Autodesk Inventor part; units mm, degrees
ref_plane "YZ Plane" through (0, 0, 0) normal (1, 0, 0) x (0, 1, 0)
ref_plane "XZ Plane" through (0, 0, 0) normal (0, 1, 0) x (-1, 0, 0)
ref_plane "XY Plane" through (0, 0, 0) normal (0, 0, 1) x (1, 0, 0)
sketch "Sketch1" plane through (0, 0, 0) normal (0, 1, 0) x (-1, 0, 0)
  line L0 (11, 19.5) -> (-11, 19.5)
  line L1 (-11, 19.5) -> (-11, -19.5)
  line L2 (-11, -19.5) -> (11, -19.5)
  line L3 (11, -19.5) -> (11, 19.5)
  line L4 (11, 19.5) -> (-11, -19.5) construction
  line L5 (-11, 19.5) -> (11, -19.5) construction
  point P0 (0, 0)
  dimension "d0" = 22
  dimension "d1" = 39
extrude "Plate1" add sketch "Sketch1" along normal blind 3
sketch "Sketch2" plane through (0, 3, 0) normal (0, 1, 0) x (1, 0, 0)
  circle A0 centre (0, -12.5) radius 2.1
  line L0 (11, -19.5) -> (11, 19.5)
  line L1 (11, 0) -> (-11, 0)
  line L2 (-11, 19.5) -> (-11, -19.5)
  circle A1 centre (0, 12.5) radius 2.1
  point P0 (0, 0)
  dimension "d3" = 4.2
  dimension "d4" = 12.5
extrude "Cut1" cut sketch "Sketch2" against normal blind 3
equation "\"d5\" = Thickness"
equation "\"d2\" = Thickness"
equation "\"BendRadius\" = Thickness"
equation "\"BendReliefWidth\" = Thickness"
equation "\"BendReliefDepth\" = 0.5 * Thickness"
equation "\"CornerReliefSize\" = 4 * Thickness"
equation "\"MinimumRemnant\" = 2 * Thickness"
equation "\"TransitionRadius\" = BendRadius"
equation "\"JacobiRadiusSize\" = BendRadius"
equation "\"GapSize\" = Thickness"
properties part number "90 graders beslag"
Check sheet for the modelled part. Datum: model origin and axes. Units: mm. Round coordinates to 2 decimals unless told otherwise and drop trailing zeros. Write each loop counter-clockwise with the first axis right and the second up, starting at its lowest first coordinate (ties: lowest second). Pieces come first, ordered by that corner, then holes. Notation, with made-up numbers: (70.5, 37) -> (82.5, 37) arc R21 ccw to (82.5, 51) -> close; hole circle Ø8 at (-8.75, -15). An arc over 180 degrees is marked (long way). Put each result on its own line as item: value.
(1) Sectioned sample at B-B (z = 12.5). Enter the section's corners in (x, y).
Values found:
outline: (-11, 0) -> (-2.1, 0) -> (-2.1, 3) -> (-11, 3) -> close; (2.1, 0) -> (11, 0) -> (11, 3) -> (2.1, 3) -> close
(2) Material ranges on line 1 (Z direction, x = 0, y = 1.6); line 2 (X direction, y = 2.7, z = -12.5); line 3 (X direction, y = 2.1, z = 11.5), recorded low to high.
Values found:
line 1: z = -19.5 to -14.6, -10.4 to 10.4, 14.6 to 19.5
line 2: x = -11 to -2.1, 2.1 to 11
line 3: x = -11 to -1.85, 1.85 to 11
(3) Mould release check, pull along X, two halves, no side actions. Record for faces 1 (the face through (-0.273, 1.521, 10.418)), 2 (the face through (11, 1, 0)), 3 (the face through (0, 1, 19.5)): released by +X, released by -X, zero draft, split by the parting line, or undercut.
Values found:
face 1: undercut
face 2: released by +X
face 3: zero draft
(4) Sectioned sample at A-A (x = 0). Enter the section's corners in (y, z).
Values found:
outline: (0, -19.5) -> (3, -19.5) -> (3, -14.6) -> (0, -14.6) -> close; (0, -10.4) -> (3, -10.4) -> (3, 10.4) -> (0, 10.4) -> close; (0, 14.6) -> (3, 14.6) -> (3, 19.5) -> (0, 19.5) -> close
(5) Sectioned sample at D-D (z = -12). Enter the section's corners in (x, y), plus the area to 3 significant figures.
Values found:
outline: (-11, 0) -> (-2.04, 0) -> (-2.04, 3) -> (-11, 3) -> close; (2.04, 0) -> (11, 0) -> (11, 3) -> (2.04, 3) -> close
area: 53.8 mm^2
(6) Sectioned sample at C-C (y = 2.55). Enter the section's corners in (x, z).
Values found:
outline: (-11, -19.5) -> (11, -19.5) -> (11, 19.5) -> (-11, 19.5) -> close; hole circle Ø4.2 at (0, -12.5); hole circle Ø4.2 at (0, 12.5)
